Geometry check sheet. Reference: the model listing, model coordinates, mm. A direction names the side the tool comes from. Give positions to 0.01 mm unless a question says otherwise; leave off trailing zeros. Loops run counter-clockwise (first coordinate to the right, second up) from the corner with the lowest first, then second, coordinate; pieces in that order, holes last. Notation, with made-up numbers: (56.5, 83.5) -> (96.5, 83.5) arc R20 cw to (96.5, 112.5) -> close; hole circle Ø8 at (34.5, 42). An arc over 180 degrees is marked (long way). One line per item, written item: value. Start each with the question number.
(1) Sectioned sample at C-C, the plane z = -28.5. Record the cut outline in (x, y), then the cut area to 3 significant figures.
(2) Tool access check on faces 1 (the face through (52.927, 7.148, -25.574)), 2 (the face through (71.826, 8.76, -23.455)), 3 (the face through (61, 9, -40.148)), 4 (the face through (54, 7, -46.839)), 5 (the face through (76, 0, -35)). Record the directions out of +Z, -Z, +X, -X, +Y, -Y that give a thin tool (end or side, any length) a straight path to the whole face; none if there is none.
(3) Scan lines: line 1 along X through (y, z) = (12, -42); line 2 along Y through (x, z) = (66, -37); line 3 along Z through (x, y) = (77.5, 7). Record each from-to range of solid material in increasing order. Write a range as from..to.
(4) Sectioned sample at B-B, the plane x = 65.5. Record the cut outline in (y, z).
(5) Sectioned sample at A-A, the plane y = 2.75. State how many separate pieces and enclosed holes the cut face has, then the cut area to 3 significant figures.
(6) Sectioned sample at D-D, the plane x = 56.5. Record the cut outline in (y, z).
(7) Draft check along X on faces 6 (the face through (56, 7, -22.751)), 7 (the face through (69.348, 9, -22)), 8 (the face through (55.82, 7, -46)). Enter one of: pulls with the +X half, pulls with the -X half, needs draft (parallel to the pull), parting line crosses it, or undercut.
(8) Gauge pin test, flat ends, axial feed: pin 1 Ø1.9 at (x, y) = (53.5, 10.5) entering from -Z; pin 2 Ø4.5 at (y, z) = (7, -44) entering from +X; pin 3 Ø1.2 at (x, y) = (71.5, 8) entering from -Z. Record the tip position at first contact, or that the pin passes through.
from build123d import *

# Parameters (mm, degrees)
BOSS_EXTRUDE1_DEPTH = 14.5
SKETCH2_R           = 2.5
CUT_EXTRUDE1_DEPTH  = 4


with BuildPart() as part:
    # Sketch1 → Boss-Extrude1 (new body)
    with BuildSketch(Plane(origin=(0, 0, 0), x_dir=(1, 0, 0), z_dir=(0, 1, 0))):
        Polygon((69.586467452, 65.357930026), (62.622760441, 65.357930026), (61.753444713, 43.538105233), (61.753444713, 40.147773891), (60.253444713, 40.147773891), (60.253444713, 44.839166535), (55.819934496, 44.839166535), (55.819934496, 46.839166535), (51.994945289, 46.839166535), (51.994945289, 37.839166535), (48.604613947, 36.361329796), (48.604613947, 27.361329796), (51.994945289, 25.839166535), (53.886066531, 25.301731423), (54.520425265, 22.751046211), (57.428168594, 22.751046211), (57.834181975, 24.179721996), (62.861391899, 22.751046211), (62.861391899, 21.357930026), (69.347835994, 21.357930026), (69.347835994, 22.751046211), (74.375045918, 24.179721996), (74.781059299, 22.751046211), (77.688802628, 22.751046211), (78.323161362, 25.301731423), (80.214282604, 25.839166535), (83.604613947, 27.361329796), (83.604613947, 36.361329796), (80.214282604, 37.839166535), (80.214282604, 46.839166535), (76.389293398, 46.839166535), (76.389293398, 44.839166535), (71.955783181, 44.839166535), (71.955783181, 40.147773891), (70.455783181, 40.147773891), (70.455783181, 43.538105233), align=None)
    extrude(amount=BOSS_EXTRUDE1_DEPTH)

    # Sketch2 → Cut-Extrude1 (cut)
    with BuildSketch(Plane(origin=(0, 0, 0), x_dir=(-1, 0, 0), z_dir=(0, -1, 0))):
        Polygon((-60.253444713, 40.147773891), (-60.347786937, 23.465384103), (-62.861391899, 22.751046211), (-62.861391899, 21.357930026), (-69.347835994, 21.357930026), (-69.347835994, 22.751046211), (-71.861440956, 23.465384103), (-71.955783181, 40.147773891), (-70.455783181, 40.147773891), (-70.455783181, 43.538105233), (-69.586467452, 65.357930026), (-62.622760441, 65.357930026), (-61.753444713, 43.538105233), (-61.753444713, 40.147773891), align=None)
        with Locations((-66.104613947, 40.807926742)):
            Circle(SKETCH2_R, mode=Mode.SUBTRACT)
    extrude(amount=-CUT_EXTRUDE1_DEPTH, mode=Mode.SUBTRACT)


solid = part.part
Calculated:
1. outline: (48.6, 0) -> (60.32, 0) -> (60.32, 4) -> (71.89, 4) -> (71.89, 0) -> (83.6, 0) -> (83.6, 14.5) -> (48.6, 14.5) -> close
1. area: 461 mm2
2. face 1: +Z, -X, +Y, -Y
2. face 2: +Z, +Y, -Y
2. face 3: -Z, +Y, -Y
2. face 4: -Z, -X, +Y, -Y
2. face 5: +Z, -Z, +X, -X, -Y
3. line 1: x = 51.99..60.25, 61.75..70.46, 71.96..80.21
3. line 2: y = 4..14.5
3. line 3: z = -46.84..-22.75
4. outline: (0, -43.23) -> (4, -43.23) -> (4, -65.36) -> (14.5, -65.36) -> (14.5, -21.36) -> (4, -21.36) -> (4, -38.38) -> (0, -38.38) -> close
5. separate pieces: 3
5. enclosed holes: 0
5. area: 454 mm2
6. outline: (0, -44.84) -> (14.5, -44.84) -> (14.5, -22.75) -> (0, -22.75) -> close
7. face 6: needs draft
7. face 7: pulls with the +X half
7. face 8: undercut
8. pin 1: stops at z = -46.84
8. pin 2: stops at x = 80.21
8. pin 3: stops at z = -44.84
